```python
from build123d import *

# Parameters (mm, degrees)
F0_W     = 12
F0_H     = 29
F0_H_2   = 4
F0_W_2   = 90
F0_H_3   = 31
F0_W_3   = 4
F1_DEPTH = 2
F2_DEPTH = 11
F3_D     = 3.5
F4_DEPTH = 3


with BuildPart() as f1:
    # F0 (on Front) → F1 (new body)
    with BuildSketch(Plane.XZ):
        with Locations((-115.3087058514, -52.4680708938)):
            Rectangle(F0_W, F0_H)
        with Locations((-115.3087058514, -35.9680708938)):
            Rectangle(F0_W, F0_H_2)
        Polygon((-109.3087058514, -66.9680708938), (-109.3087058514, -70.9680708938), (-1.3087058514, -70.9680708938), (-1.3087058514, -66.9680708938), (-1.3087058514, -37.9680708938), (-1.3087058514, -33.9680708938), (-109.3087058514, -33.9680708938), (-109.3087058514, -37.9680708938), align=None)
        with Locations((-54.3087058514, -52.4680708938)):
            Rectangle(F0_W_2, F0_H_3, mode=Mode.SUBTRACT)
        with Locations((-115.3087058514, -68.9680708938)):
            Rectangle(F0_W, F0_H_2)
        with Locations((0.6912941486, -35.9680708938)):
            Rectangle(F0_W_3, F0_H_2)
        with Locations((0.6912941486, -52.4680708938)):
            Rectangle(F0_W_3, F0_H)
        with Locations((0.6912941486, -68.9680708938)):
            Rectangle(F0_W_3, F0_H_2)
    extrude(amount=F1_DEPTH)

    # F0 (on Front) → F2 (join)
    with BuildSketch(Plane.XZ):
        with Locations((-54.3087058514, -52.4680708938)):
            Rectangle(F0_W_2, F0_H_3)
    extrude(amount=F2_DEPTH)

    # F3 (through all)
    with Locations(Plane(origin=(0, 0, 0), x_dir=(1, 0, 0), z_dir=(0, 1, 0))):
        with Locations((-109.3087058514, 37.9680708938), (-109.3087058514, 66.9680708938), (-1.3087058514, 37.9680708938), (-1.3087058514, 66.9680708938)):
            Hole(F3_D / 2)

    # F0 (on Front) → F4 (join)
    with BuildSketch(Plane.XZ):
        with Locations((-54.3087058514, -52.4680708938)):
            Rectangle(F0_W_2, F0_H_3)
    extrude(amount=-F4_DEPTH)


solid = f1.part
```
The model under review builds one solid part; all positions refer to its coordinate system, in mm. A direction names the side the tool comes from. Round coordinates to 2 decimals unless told otherwise and drop trailing zeros. Loops run counter-clockwise (first coordinate to the right, second up) from the corner with the lowest first, then second, coordinate; pieces in that order, holes last.
Item 1: For faces 1 (the face through (-99.309, -6, -53)), 2 (the face through (2.691, -1, -53)), 3 (the face through (-55, -6, -36.968)), 4 (the face through (-55, 1, -36.968)), list the 3-axis set-ups (+Z, -Z, +X, -X, +Y, -Y) from which the entire face can be reached by the end or side of a thin tool; tool diameter is ignored.
Determined:
face 1: +Z, -Z, -X, -Y
face 2: +Z, -Z, +X, +Y, -Y
face 3: +Z, +X, -X, -Y
face 4: +Z, +X, -X, +Y
Item 2: Take a section at A-A (z = -44.5). Write out the cut boundary in (x, y).
Determined:
outline: (-121.31, -2) - (-99.31, -2) - (-99.31, -11) - (-9.31, -11) - (-9.31, -2) - (2.69, -2) - (2.69, 0) - (-9.31, 0) - (-9.31, 3) - (-99.31, 3) - (-99.31, 0) - (-121.31, 0) - close
Item 3: Take a section at D-D (x = -6.5). Write out the cut boundary in (y, z).
Determined:
outline: (-2, -70.97) - (0, -70.97) - (0, -33.97) - (-2, -33.97) - close
Item 4: Take a section at B-B (x = -26). Write out the cut boundary in (y, z), then the cut area to 3 significant figures.
Determined:
outline: (-11, -67.97) - (-2, -67.97) - (-2, -70.97) - (0, -70.97) - (0, -67.97) - (3, -67.97) - (3, -36.97) - (0, -36.97) - (0, -33.97) - (-2, -33.97) - (-2, -36.97) - (-11, -36.97) - close
area: 446 mm2
Item 5: For line 1 (Y direction, x = -72.5, z = -68.5); line 2 (Z direction, x = -17.5, y = -4); line 3 (X direction, y = -3, z = -43), list the stretches that pass through material, from the lowest coordinate up.
Determined:
line 1: y = -2 to 0
line 2: z = -67.97 to -36.97
line 3: x = -99.31 to -9.31
Item 6: Mouldability with a two-part tool opening along X and no side actions: class faces 5 (the face through (-55, 1, -67.968)), 6 (the face through (-99.309, 1, -53)), 7 (the face through (-9.309, -6, -53)), 8 (the face through (-1.081, -1.014, -68.703)) as released by +X, released by -X, zero draft, split by the parting line, or undercut.
Determined:
face 5: zero draft
face 6: released by -X
face 7: released by +X
face 8: undercut
Item 7: Take a section at C-C (y = -9.75). Write out the cut boundary in (x, z).
Determined:
outline: (-99.31, -67.97) - (-9.31, -67.97) - (-9.31, -36.97) - (-99.31, -36.97) - close
Item 8: Clearance check with flat-ended pins moving along their axes: pin 1 Ø3 at (y, z) = (-5.5, -53.5) entering from -X; pin 2 Ø4.5 at (x, y) = (-72, -5.5) entering from +Z; pin 3 Ø5.5 at (x, z) = (-109.31, -66.97) entering from -Y. State where each tip first meets the part, or that it passes through.
Determined:
pin 1: stops at x = -99.31
pin 2: stops at z = -36.97
pin 3: stops at y = -2
